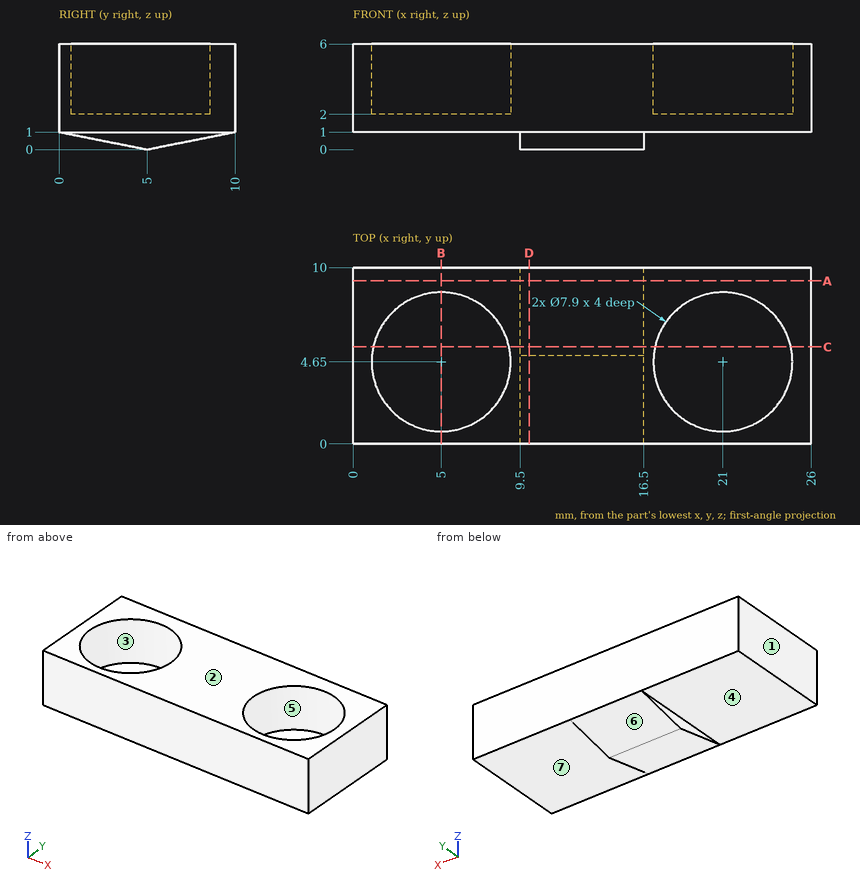
For this review, use the dimensioned drawing (mm, ordinates from the lowest corner) and the shaded views. A direction names the side the tool comes from. Round coordinates to 2 decimals unless told otherwise and drop trailing zeros. Write each loop counter-clockwise with the first axis right and the second up, starting at its lowest first coordinate (ties: lowest second). Pieces come first, ordered by that corner, then holes. Notation, with made-up numbers: (79, 46.25) - (96, 46.25) arc R22 cw to (96, 62.25) - close; hole circle Ø10 at (-28.5, 83.5). An arc over 180 degrees is marked (long way). One line per item, written item: value. Start each with the question number.
1. Clearance check with flat-ended pins moving along their axes: P1, Ø4, axis at x = 3.5, y = 3, coming from the +Z side; P2, Ø3, axis at x = 22.5, y = 2.5, coming from the -Z side. State where each tip first meets the part, or that it passes through.
2. Consider section C-C on y = 5.5. Write out the cut boundary in (x, z).
3. Consider section B-B on x = 5. Write out the cut boundary in (y, z).
4. Consider section D-D on x = 10. Write out the cut boundary in (y, z), and give its area (3 significant figures).
5. The part is to be moulded in two halves that separate along X. For the marked faces 1, 2 and 3, say which applies: released by +X, released by -X, zero draft, split by the parting line, or undercut.
6. Machinability: for the marked faces 4, 5, 6 and 7, which of the approach directions +Z, -Z, +X, -X, +Y, -Y give a long, thin tool a straight path to every point of the face, cutting with its end or side? Answer none if there is none.
7. Consider section A-A on y = 9.25. Write out the cut boundary in (x, z), and give its area (3 significant figures).
8. To check wall thickness, follow L1, parallel to Y at x = 5, z = 4.9; L2, parallel to X at y = 1, z = 4.75; L3, parallel to X at y = 3.75, z = 5. State the ranges of each line that lie inside material, in increasing order. Write a range as from..to.
Checks:
1. P1: stops at z = 6
1. P2: stops at z = 1
2. outline: (0, 1) - (9.5, 1) - (9.5, 0.1) - (16.5, 0.1) - (16.5, 1) - (26, 1) - (26, 6) - (24.86, 6) - (24.86, 2) - (17.14, 2) - (17.14, 6) - (8.86, 6) - (8.86, 2) - (1.14, 2) - (1.14, 6) - (0, 6) - close
3. outline: (0, 1) - (10, 1) - (10, 6) - (8.6, 6) - (8.6, 2) - (0.7, 2) - (0.7, 6) - (0, 6) - close
4. outline: (0, 1) - (5, 0) - (10, 1) - (10, 6) - (0, 6) - close
4. area: 55.0 mm^2
5. face 1: released by -X
5. face 2: zero draft
5. face 3: undercut
6. face 4: -Z, -X, +Y, -Y
6. face 5: +Z
6. face 6: -Z, +X, -X, +Y
6. face 7: -Z, +X, +Y, -Y
7. outline: (0, 1) - (9.5, 1) - (9.5, 0.85) - (16.5, 0.85) - (16.5, 1) - (26, 1) - (26, 6) - (0, 6) - close
7. area: 131 mm^2
8. L1: y = 0..0.7, 8.6..10
8. L2: x = 0..3.49, 6.51..19.49, 22.51..26
8. L3: x = 0..1.15, 8.85..17.15, 24.85..26
